Model file for the job. Use its own axes, mm. Face numbers are marked on the shaded views. A direction names the side the tool comes from. Round coordinates to 2 decimals unless told otherwise and drop trailing zeros. Loops run counter-clockwise (first coordinate to the right, second up) from the corner with the lowest first, then second, coordinate; pieces in that order, holes last. Notation, with made-up numbers: M 12.25,28.25 L 32.25,28.25 A9 ccw 32.25,45.25 Z; hole C 51.5,1.25 d3. An arc over 180 degrees is marked long. Answer in a Markdown table with one row per item.
from build123d import *
from OCP.BRepFilletAPI import BRepFilletAPI_MakeChamfer

# Parameters (mm, degrees)
BOSS_EXTRU_1_DEPTH      = 2
BOSS_EXTRU_2_DEPTH      = 20
ESQUISSE2_R             = 1.4
ENL_V_MAT_EXTRU_1_DEPTH = 75.296702484
CHANFREIN1_SIZE         = 15
CHANFREIN1_SIZE_2       = 20


with BuildPart() as part:
    # Esquisse1 → Boss.-Extru.1 (new body)
    with BuildSketch(Plane.XY):
        Polygon((0, 0), (43.5, 0), (44.5, 0), (44.5, 2.018181818), (43.5, 2.018181818), (43.5, 4), (48.5, 4), (48.5, 2), (47.5, 2), (47.5, 0), (48.5, 0), (64, 0), (64, 32), (0, 32), (0, 19.5), (2, 19.5), (2, 20.5), (4, 20.5), (4, 15.5), (2, 15.5), (2, 16.5), (0, 16.5), (0, 13.5), align=None)
    extrude(amount=BOSS_EXTRU_1_DEPTH)

    # Esquisse3 → Boss.-Extru.2 (add)
    with BuildSketch(Plane.XY.offset(2)):
        Polygon((26.917717359, 32), (29.417717359, 32), (48.5, 32), (48.5, 30), (33.5, 30), (33.5, 0), (31, 0), (31, 30), (16, 30), (16, 32), align=None)
    extrude(amount=BOSS_EXTRU_2_DEPTH)

    # Esquisse2 → Enlèv. mat.-Extru.1 (cut, through all)
    with BuildSketch(Plane.XY.offset(2)):
        with Locations((8, 18)):
            Circle(ESQUISSE2_R)
        with Locations((28, 18)):
            Circle(ESQUISSE2_R)
        with Locations((46, 28)):
            Circle(ESQUISSE2_R)
        with Locations((46, 8)):
            Circle(ESQUISSE2_R)
    extrude(amount=-ENL_V_MAT_EXTRU_1_DEPTH, mode=Mode.SUBTRACT)

    # Chanfrein1
    chanfrein1_edges_1 = [part.edges().sort_by_distance(p)[0] for p in [
        (48.5, 31, 22),
    ]]
    chanfrein1_side_1 = [part.faces().sort_by_distance(p)[0] for p in [
        (48.2, 31, 22),
    ]]
    chanfrein1_edges_2 = [part.edges().sort_by_distance(p)[0] for p in [
        (16, 31, 22),
    ]]
    chanfrein1_side_2 = [part.faces().sort_by_distance(p)[0] for p in [
        (16.3, 31, 22),
    ]]
    chanfrein1 = BRepFilletAPI_MakeChamfer(part.part.solid().wrapped)
    for e in chanfrein1_edges_1:
        chanfrein1.Add(CHANFREIN1_SIZE - 0.0001, CHANFREIN1_SIZE_2 - 0.0001, e.wrapped, chanfrein1_side_1[0].wrapped)
    for e in chanfrein1_edges_2:
        chanfrein1.Add(CHANFREIN1_SIZE - 0.0001, CHANFREIN1_SIZE_2 - 0.0001, e.wrapped, chanfrein1_side_2[0].wrapped)
    add(Compound.cast(chanfrein1.Shape()), mode=Mode.REPLACE)  # a hair under: the kernel refuses the full size


solid = part.part
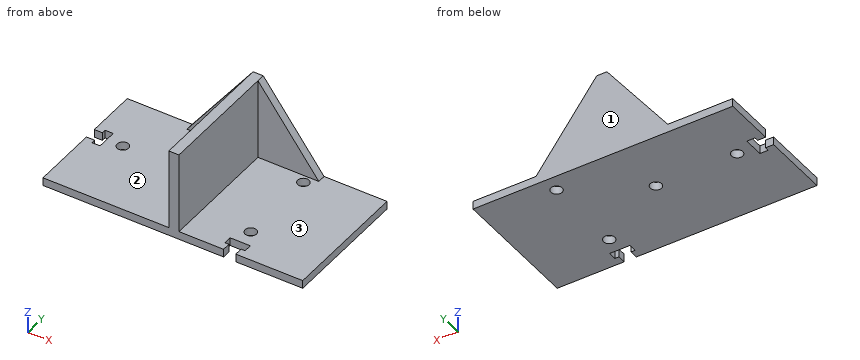
1. Wall check: probe 1 along Y at (x, z) = (46, 0.9); probe 2 along Y at (x, z) = (8, 0.95); probe 3 along X at (y, z) = (29.5, 12). Give the ranges that are in metal, low to high.
Verdict:
| item | result |
|---|---|
| probe 1 | y = 4 to 6.6, 9.4 to 26.6, 29.4 to 32 |
| probe 2 | y = 0 to 16.6, 19.4 to 32 |
| probe 3 | x = 31 to 33.5 |
2. Saw through at D-D (z = 7.75). Write the cut outline in (x, y).
Verdict:
| item | result |
|---|---|
| outline | M 20.31,30 L 31,30 L 31,0 L 33.5,0 L 33.5,30 L 44.19,30 L 44.19,32 L 20.31,32 Z |
3. Saw through at B-B (y = 8). Write the cut outline in (x, z).
Verdict:
| item | result |
|---|---|
| outline | M 0,0 L 44.6,0 L 44.6,2 L 33.5,2 L 33.5,22 L 31,22 L 31,2 L 0,2 Z; M 47.4,0 L 64,0 L 64,2 L 47.4,2 Z |
4. Saw through at A-A (x = 8). Write the cut outline in (y, z).
Verdict:
| item | result |
|---|---|
| outline | M 0,0 L 16.6,0 L 16.6,2 L 0,2 Z; M 19.4,0 L 32,0 L 32,2 L 19.4,2 Z |
5. Saw through at C-C (y = 18). Write the cut outline in (x, z), and give its area (3 significant figures).
Verdict:
| item | result |
|---|---|
| outline | M 4,0 L 6.6,0 L 6.6,2 L 4,2 Z; M 9.4,0 L 26.6,0 L 26.6,2 L 9.4,2 Z; M 29.4,0 L 64,0 L 64,2 L 33.5,2 L 33.5,22 L 31,22 L 31,2 L 29.4,2 Z |
| area | 159 mm² |
6. Tool access for the marked faces 1, 2 and 3: list every direction of +Z, -Z, +X, -X, +Y, -Y with a clear straight run to the whole face (end or side of a thin tool).
Verdict:
| item | result |
|---|---|
| face 1 | +Z, -Z, +X, -X, +Y |
| face 2 | +Z, -X, -Y |
| face 3 | +Z, +X, -Y |
7. Pin check, flat tips, straight feed: pin 1 (3 mm diameter, centred on x = 8, y = 18, fed in from +Z); pin 2 (2 mm diameter, centred on y = 22.5, z = 10, fed in from +X); pin 3 (2 mm diameter, centred on x = 23, z = 8, fed in from -Y). Stop position of each tip, or through.
Verdict:
| item | result |
|---|---|
| pin 1 | stops at z = 2 |
| pin 2 | stops at x = 33.5 |
| pin 3 | stops at y = 30 |
